The model under review builds one solid part; all positions refer to its coordinate system, in mm. A direction names the side the tool comes from. Give positions to 0.01 mm unless a question says otherwise; leave off trailing zeros. Order: outer loops, then holes, each group sorted by start corner. A loop starts at its lowest first (then second) coordinate and runs counter-clockwise, first axis right, second up. Notation, with made-up numbers: (69, -2) - (114, -2) arc R29 ccw to (114, 35) - close; hole circle Ø9 at (-10.75, -27.5). An arc over 180 degrees is marked (long way). Use CSV: the item, a comma, the result in double quotes.
```python
from build123d import *

# Parameters (mm, degrees)
SKETCH1_W           = 56
SKETCH1_H           = 18
LOUVER_FLAP_DEPTH   = 1
SKETCH2_R           = 1.5
PIVOT_SHAFT_L_DEPTH = 5
PIVOT_SHAFT_R_START = 5
SKETCH3_R           = 1.5
PIVOT_SHAFT_R_DEPTH = 5
CRANK_ARM_DEPTH     = 2
SKETCH5_R           = 1.25
CRANK_PIN_DEPTH     = 4


with BuildPart() as part:
    # Sketch1 → Louver_Flap (new, symmetric)
    with BuildSketch(Plane.XY):
        Rectangle(SKETCH1_W, SKETCH1_H)
    extrude(amount=LOUVER_FLAP_DEPTH, both=True)

    # Sketch2 → Pivot_Shaft_L (add)
    with BuildSketch(Plane.ZY.offset(28)):
        with Locations(Location((0, 0, 0), (0, 0, 131.810314896))):
            Circle(SKETCH2_R)
    extrude(amount=PIVOT_SHAFT_L_DEPTH)

    # Sketch3 → Pivot_Shaft_R (add)
    with BuildSketch(Plane(origin=(28, 0, 0), x_dir=(0, 0, -1), z_dir=(1, 0, 0)).offset(PIVOT_SHAFT_R_START)):
        with Locations(Location((0, 0, 0), (0, 0, 48.189685104))):
            Circle(SKETCH3_R)
    extrude(amount=-PIVOT_SHAFT_R_DEPTH)

    # Sketch4 → Crank_Arm (add)
    with BuildSketch(Plane(origin=(33, 0, 0), x_dir=(0, 0, -1), z_dir=(1, 0, 0))):
        Polygon((-3.522080132, -0.308142084), (8.650417232, -10.522080132), (11.86435528, -6.691857916), (-0.308142084, 3.522080132), align=None)
    extrude(amount=CRANK_ARM_DEPTH)

    # Sketch5 → Crank_Pin (add)
    with BuildSketch(Plane(origin=(35, 0, 0), x_dir=(0, 0, -1), z_dir=(1, 0, 0))):
        with Locations((8.342275148, -7)):
            Circle(SKETCH5_R)
    extrude(amount=CRANK_PIN_DEPTH)


solid = part.part
```
Item 1: Mouldability with a two-part tool opening along X and no side actions: class faces 1 (the face through (-30.46, 0.73, 1.31)), 2 (the face through (30.535, 1.367, -0.618)), 3 (the face through (39, -7, -8)) as pulls with the +X half, pulls with the -X half, needs draft (parallel to the pull), parting line crosses it, or undercut.
Results list:
face 1,"needs draft"
face 2,"undercut"
face 3,"pulls with the +X half"
Item 2: Take a section at B-B, the plane x = 1. Give the boundary of the cut face in (y, z).
Results list:
outline,"(-9, -1) - (9, -1) - (9, 1) - (-9, 1) - close"
Item 3: Tool access review of faces 4 (the face through (33.986, 1.634, 1.893)), 5 (the face through (33.986, -8.634, -10.235)), 6 (the face through (36.972, -6.945, -7.093)): name each direction out of +Z, -Z, +X, -X, +Y, -Y from which nothing blocks a thin tool from reaching the whole face with its end or side.
Results list:
face 4,"+Z, +X, +Y"
face 5,"-Z, +X, -X, -Y"
face 6,"+X"
Item 4: Take a section at A-A, the plane y = -3. Give the boundary of the cut face in (x, z).
Results list:
outline,"(-28, -1) - (28, -1) - (28, 1) - (-28, 1) - close; (33, -7.46) - (35, -7.46) - (35, 0.31) - (33, 0.31) - close"
Item 5: Clearance check with flat-ended pins moving along their axes: pin 1 (5 mm diameter, centred on y = -8.5, z = -9.5, fed in from -X); pin 2 (3 mm diameter, centred on y = -3, z = -0.5, fed in from +X); pin 3 (6 mm diameter, centred on x = 7.5, z = -2, fed in from -Y). State where each tip first meets the part, or that it passes through.
Results list:
pin 1,"stops at x = 33"
pin 2,"stops at x = 35"
pin 3,"stops at y = -9"
Item 6: Wall thickness on L1, parallel to X at y = -8.5, z = -9.25; L2, parallel to Z at x = -17.5, y = -3.5; L3, parallel to X at y = -6.5, z = -8.75: over which ranges is each line inside the solid? List them lowest first.
Results list:
L1,"x = 33 to 35"
L2,"z = -1 to 1"
L3,"x = 33 to 39"
